Model file for the job. Use its own axes, mm. A direction names the side the tool comes from. Coordinates: 2 decimals unless noted, no trailing zeros. Write each loop counter-clockwise with the first axis right and the second up, starting at its lowest first coordinate (ties: lowest second). Pieces come first, ordered by that corner, then holes. Notation, with made-up numbers: (68, -32) - (109, -32) arc R28 cw to (109, -10) - close; hole circle Ø6 at (87.25, -30). An arc over 180 degrees is marked (long way). Put each result on its own line as item: value. Start each with the question number.
1. Which spindle directions (+Z, -Z, +X, -X, +Y, -Y) get a long thin tool onto all of the face, cutting with end or side? Do faces 4 (the face through (8.57, -69.74, 1.48)), 5 (the face through (-75.303, 49.14, 1.521)), 6 (the face through (-75.504, -49.341, 1.521)). Say none if no direction does.
2. Drop flat-ended pins along their axis: P1, Ø0.9, axis at x = -68.5, z = 2, coming from the +Y side; P2, Ø0.9, axis at x = 64, z = 1.5, coming from the +Y side; P3, Ø1.5, axis at x = -66, z = 2, coming from the -Y side. Give the stop position or say it passes through.
3. Saw through at A-A, the plane y = -3.5. Write the cut outline in (x, z), plus the area to 3 significant figures.
4. Pull direction X, two halves, no side cores. Call faces 1 (the face through (0.839, 99.996, 1.479)), 2 (the face through (49.14, 75.303, 1.521)), 3 (the face through (8.5, -76.81, 1.48)): released by +X, released by -X, zero draft, split by the parting line, or undercut.
5. Saw through at B-B, the plane z = 2.25. Give the number of separate pieces and of enclosed holes in the cut face, plus the area to 3 significant figures.
6. Saw through at D-D, the plane x = 39.5. Write the cut outline in (y, z).
7. Drill centre lines: L1, parallel to X at y = -73, z = 2.15; L2, parallel to X at y = 54.5, z = 2.1; L3, parallel to Y at x = -48, z = 0.4. Where is each one in solid material? Low to high. Write a range as from..to.
8. Saw through at C-C, the plane x = -60. Write the cut outline in (y, z), plus the area to 3 significant figures.
```python
from build123d import *

# Parameters (mm, degrees)
CROQUIS1_R              = 100
SALIENTE_EXTRUIR1_DEPTH = 3
CROQUIS3_R              = 110
CORTAR_EXTRUIR1_DEPTH   = 3
REDONDEO1_R             = 10
CORTAR_EXTRUIR2_DEPTH   = 142.453172607
CROQUIS6_W              = 10
CROQUIS6_H              = 15
CROQUIS6_W_2            = 20
CROQUIS6_H_2            = 10
CROQUIS6_W_3            = 15
CROQUIS6_H_3            = 8
CORTAR_EXTRUIR4_DEPTH   = 10
REDONDEO3_R             = 5


with BuildPart() as part:
    # Croquis1 → Saliente-Extruir1 (new body)
    with BuildSketch(Plane.XY):
        Circle(CROQUIS1_R)
    extrude(amount=SALIENTE_EXTRUIR1_DEPTH)

    # Croquis3 → Cortar-Extruir1 (cut)
    with BuildSketch(Plane.XY.offset(3)):
        with Locations((190, 0)):
            Circle(CROQUIS3_R)
    extrude(amount=-CORTAR_EXTRUIR1_DEPTH, mode=Mode.SUBTRACT)

    # Redondeo1
    redondeo1_edges = [part.edges().sort_by_distance(p)[0] for p in [
        (89.473684211, -44.659375654, 1.5),
        (89.473684211, 44.659375654, 1.5),
    ]]
    fillet(redondeo1_edges, radius=REDONDEO1_R)

    # Croquis4 → Cortar-Extruir2 (cut, through all)
    with BuildSketch(Plane.XY.offset(3)):
        Polygon((-57.629202667, -83.792153571), (-83.792153571, -57.629202667), (-68.235804385, -42.072853481), (-42.072853481, -68.235804385), align=None)
        Polygon((-57.629202667, 83.792153571), (-42.072853481, 68.235804385), (-68.235804385, 42.072853481), (-83.792153571, 57.629202667), align=None)
        Polygon((83.792153571, 57.629202667), (68.235804385, 42.072853481), (42.072853481, 68.235804385), (57.629202667, 83.792153571), align=None)
        Polygon((57.629202667, -83.792153571), (42.072853481, -68.235804385), (68.235804385, -42.072853481), (83.792153571, -57.629202667), align=None)
    extrude(amount=-CORTAR_EXTRUIR2_DEPTH, mode=Mode.SUBTRACT)

    # Croquis6 → Cortar-Extruir4 (cut)
    with BuildSketch(Plane.XY.offset(3)):
        with Locations((63.24, 0)):
            Rectangle(CROQUIS6_W, CROQUIS6_H)
        with Locations((-68.235804385, 0)):
            Rectangle(CROQUIS6_W, CROQUIS6_H)
        with Locations((0, 73.24)):
            Rectangle(CROQUIS6_W_2, CROQUIS6_H_2)
        with Locations((0, -73.24)):
            Rectangle(CROQUIS6_W_2, CROQUIS6_H_2)
        with Locations((0, -90.24)):
            Rectangle(CROQUIS6_W_3, CROQUIS6_H_3)
    extrude(amount=-CORTAR_EXTRUIR4_DEPTH, mode=Mode.SUBTRACT)

    # Redondeo3
    redondeo3_edges = [part.edges().sort_by_distance(p)[0] for p in [
        (10, 68.24, 1.5),
        (-10, 68.24, 1.5),
        (10, 78.24, 1.5),
        (-10, 78.24, 1.5),
        (10, -78.24, 1.5),
        (-10, -78.24, 1.5),
        (10, -68.24, 1.5),
        (-10, -68.24, 1.5),
    ]]
    fillet(redondeo3_edges, radius=REDONDEO3_R - 0.0001)  # a hair under: the kernel refuses the full size


solid = part.part
```
Final values:
1. face 4: +Z, -Z
1. face 5: +Z, -Z, +Y
1. face 6: +Z, -Z, -Y
2. P1: stops at y = 42.79
2. P2: stops at y = 46.76
2. P3: stops at y = -45.06
3. outline: (-99.94, 0) - (-73.24, 0) - (-73.24, 3) - (-99.94, 3) - close; (-63.24, 0) - (58.24, 0) - (58.24, 3) - (-63.24, 3) - close; (68.24, 0) - (80.06, 0) - (80.06, 3) - (68.24, 3) - close
3. area: 480 mm²
4. face 1: split by the parting line
4. face 2: released by +X
4. face 3: undercut
5. separate pieces: 1
5. enclosed holes: 5
5. area: 26,300 mm²
6. outline: (-91.87, 0) - (91.87, 0) - (91.87, 3) - (-91.87, 3) - close
7. L1: x = -46.84..-9.99, 9.99..46.84
7. L2: x = -83.84..-80.66, -55.81..55.81, 80.66..83.84
7. L3: y = -87.73..-74.16, -62.31..62.31, 74.16..87.73
8. outline: (-50.31, 0) - (50.31, 0) - (50.31, 3) - (-50.31, 3) - close
8. area: 302 mm²
